Source: CAD feature listing. Evaluate the final solid. Frame: model axes, mm. Face numbers are marked on the shaded views. A direction names the side the tool comes from. Give positions to 0.01 mm unless a question says otherwise; leave off trailing zeros. Loops run counter-clockwise (first coordinate to the right, second up) from the corner with the lowest first, then second, coordinate; pieces in that order, holes last.
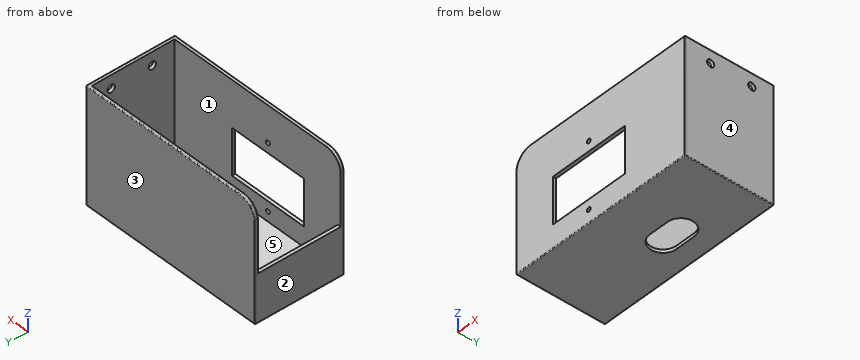
from build123d import *

# Parameters (mm, degrees)
CROQUIS1_W                          = 115
CROQUIS1_H                          = 70
SALIENTE_EXTRUIR1_DEPTH             = 54
CORTAR_EXTRUIR1_DEPTH               = 50
CROQUIS3_W                          = 49
CROQUIS3_H                          = 28
CORTAR_EXTRUIR2_DEPTH               = 105.452142151
CORTAR_EXTRUIR3_DEPTH               = 95.526451324
DI_METRO_DE_TALADRO_4_5_4_5_1_D     = 4.5
DI_METRO_DE_TALADRO_4_5_4_5_1_DEPTH = 115
DI_METRO_DE_TALADRO_2_6_2_6_1_D     = 2.6
DI_METRO_DE_TALADRO_2_6_2_6_1_DEPTH = 2
REDONDEO1_R                         = 10
REDONDEO2_R                         = 0.5


with BuildPart() as part:
    # Croquis1 → Saliente-Extruir1 (new body)
    with BuildSketch(Plane.XZ.offset(27)):
        with Locations((0, 35)):
            Rectangle(CROQUIS1_W, CROQUIS1_H)
    extrude(amount=-SALIENTE_EXTRUIR1_DEPTH)

    # Croquis2 → Cortar-Extruir1 (cut)
    with BuildSketch(Plane(origin=(0, 25, 0), x_dir=(1, 0, 0), z_dir=(0, 1, 0))):
        Polygon((-57.5, -29), (-57.5, -70), (55.5, -70), (55.5, -2), (-55.5, -2), (-55.5, -29), align=None)
    extrude(amount=-CORTAR_EXTRUIR1_DEPTH, mode=Mode.SUBTRACT)

    # Croquis3 → Cortar-Extruir2 (cut, through all)
    with BuildSketch(Plane(origin=(0, -25, 0), x_dir=(-1, 0, 0), z_dir=(0, 1, 0))):
        with Locations((8, 28)):
            Rectangle(CROQUIS3_W, CROQUIS3_H)
    extrude(amount=-CORTAR_EXTRUIR2_DEPTH, mode=Mode.SUBTRACT)

    # Croquis4 → Cortar-Extruir3 (cut, through all)
    with BuildSketch(Plane(origin=(0, 0, 0), x_dir=(-1, 0, 0), z_dir=(0, 0, -1))):
        with BuildLine():
            Line((-4.5, 15), (-16.5, 15))
            ThreePointArc((-16.5, 15), (-24.5, 7), (-16.5, -1))
            Line((-16.5, -1), (-4.5, -1))
            ThreePointArc((-4.5, -1), (3.5, 7), (-4.5, 15))
        make_face()
    extrude(amount=-CORTAR_EXTRUIR3_DEPTH, mode=Mode.SUBTRACT)

    # Diámetro de taladro Ø4.5 (4.5)1
    with Locations(Plane(origin=(57.5, 0, 0), x_dir=(0, 0, -1), z_dir=(1, 0, 0))):
        with Locations((-62, -11.5), (-62, 13.5)):
            Hole(DI_METRO_DE_TALADRO_4_5_4_5_1_D / 2, depth=DI_METRO_DE_TALADRO_4_5_4_5_1_DEPTH)

    # Diámetro de taladro Ø2.6 (2.6)1
    with Locations(Plane(origin=(0, -27, 0), x_dir=(-1, 0, 0), z_dir=(0, -1, 0))):
        with Locations((8, -48), (8, -8)):
            Hole(DI_METRO_DE_TALADRO_2_6_2_6_1_D / 2, depth=DI_METRO_DE_TALADRO_2_6_2_6_1_DEPTH)

    # Redondeo1
    redondeo1_edges = [part.edges().sort_by_distance(p)[0] for p in [
        (-57.5, -26, 70),
        (-57.5, 26, 70),
    ]]
    fillet(redondeo1_edges, radius=REDONDEO1_R)

    # Redondeo2
    redondeo2_edges = [part.edges().sort_by_distance(p)[0] for p in [
        (57.5, 27, 35),
        (5, 27, 70),
        (-57.5, 25, 44.5),
        (5, -27, 70),
        (57.5, -27, 35),
        (0, -27, 0),
        (57.5, 0, 70),
        (57.5, 0, 0),
        (-57.5, 0, 0),
        (0, 27, 0),
        (4, 25, 70),
        (-54.571067812, 25, 67.071067812),
        (-57.5, 27, 30),
        (-57.5, -27, 30),
        (-54.571067812, 27, 67.071067812),
        (-54.571067812, -27, 67.071067812),
    ]]
    fillet(redondeo2_edges, radius=REDONDEO2_R)


solid = part.part
1) Ray query, probe 1 along Y at (x, z) = (56.95, 62); probe 2 along X at (y, z) = (-26.25, 48); probe 3 along X at (y, z) = (-20, 20). Return the intervals inside material, ascending.
Checks:
probe 1: y = -27 to -13.75, -9.25 to 11.25, 15.75 to 27
probe 2: x = -57.5 to -9.3, -6.7 to 57.5
probe 3: x = -57.5 to -55.5, 55.5 to 57.5
2) Cut plane A-A (z = 48). Return loops of the section in (x, y), and give its area (3 significant figures).
Checks:
outline: (-57.5, -26.5) arc R0.5 ccw to (-57, -27) - (-9.3, -27) - (-9.3, -25) - (-57.5, -25) - close; (-57.5, 25.5) arc R0.5 ccw to (-57, 25) - (55.5, 25) - (55.5, -25) - (-6.7, -25) - (-6.7, -27) - (57, -27) arc R0.5 ccw to (57.5, -26.5) - (57.5, 26.5) arc R0.5 ccw to (57, 27) - (-57, 27) arc R0.5 ccw to (-57.5, 26.5) - close
area: 555 mm2
3) Pull-direction query (X, two-part tool) for the marked faces 3, 4 and 5; classes: released by +X, released by -X, zero draft, split by the parting line, or undercut.
Checks:
face 3: zero draft
face 4: released by +X
face 5: undercut
4) Cut plane C-C (z = 17). Return loops of the section in (x, y), and give its area (3 significant figures).
Checks:
outline: (-57.5, -26.5) arc R0.5 ccw to (-57, -27) - (-32.5, -27) - (-32.5, -25) - (-55.5, -25) - (-55.5, 25) - (55.5, 25) - (55.5, -25) - (16.5, -25) - (16.5, -27) - (57, -27) arc R0.5 ccw to (57.5, -26.5) - (57.5, 26.5) arc R0.5 ccw to (57, 27) - (-57, 27) arc R0.5 ccw to (-57.5, 26.5) - close
area: 562 mm2
5) Cut plane D-D (y = 19.5). Return loops of the section in (x, z).
Checks:
outline: (-57.5, 0.5) arc R0.5 ccw to (-57, 0) - (57, 0) arc R0.5 ccw to (57.5, 0.5) - (57.5, 69.5) arc R0.5 ccw to (57, 70) - (55.5, 70) - (55.5, 2) - (-55.5, 2) - (-55.5, 29) - (-57.5, 29) - close
6) Cut plane B-B (x = -16.5). Return loops of the section in (y, z).
Checks:
outline: (-27, 0.5) arc R0.5 ccw to (-26.5, 0) - (26.5, 0) arc R0.5 ccw to (27, 0.5) - (27, 69.5) arc R0.5 ccw to (26.5, 70) - (25.5, 70) arc R0.5 ccw to (25, 69.5) - (25, 2) - (-25, 2) - (-25, 14) - (-27, 14) - close; (-27, 42) - (-25, 42) - (-25, 70) - (-26.5, 70) arc R0.5 ccw to (-27, 69.5) - close
7) Reachability of the marked faces 1 and 2 from +Z, -Z, +X, -X, +Y, -Y: full face, straight path, thin tool, end or side. Return the list, or none.
Checks:
face 1: +Z
face 2: +Z, -Z, -X, +Y, -Y
8) Contact query for flat-ended pins moving along their axis: P1, Ø7, axis at y = 13.5, z = 62, coming from the -X side; P2, Ø8, axis at x = -4.5, y = -10.5, coming from the +Z side; P3, Ø3.5, axis at y = -11.5, z = 62, coming from the +X side. Output: stop coordinate, or through.
Checks:
P1: stops at x = 55.5
P2: stops at z = 2
P3: passes through
